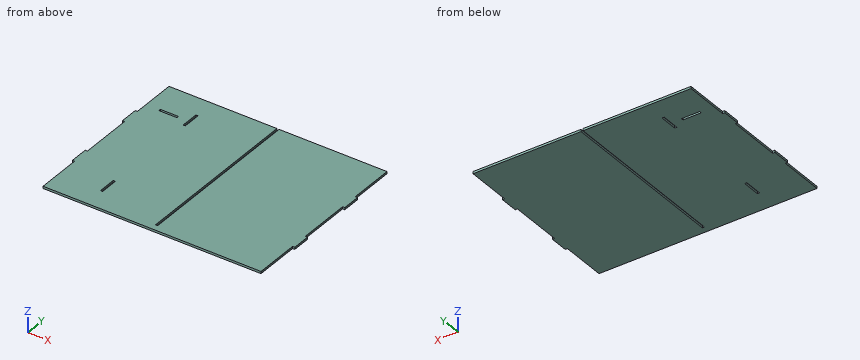
```python
from build123d import *

# Parameters (mm, degrees)
SKETCH1_W           = 6
SKETCH1_H           = 50
SKETCH1_W_2         = 50
SKETCH1_H_2         = 6
BOSS_EXTRUDE1_DEPTH = 6


with BuildPart() as part:
    # Sketch1 → Boss-Extrude1 (new body)
    with BuildSketch(Plane.XY):
        Polygon((0, 0), (297, 0), (297, -476), (303, -476), (303, 0), (600, 0), (600, -124), (606, -124), (606, -174), (600, -174), (600, -320), (606, -320), (606, -370), (600, -370), (600, -494), (0, -494), (0, -370), (-6, -370), (-6, -320), (0, -320), (0, -174), (-6, -174), (-6, -124), (0, -124), align=None)
        with Locations((119, -409)):
            Rectangle(SKETCH1_W, SKETCH1_H, mode=Mode.SUBTRACT)
        with Locations((119, -85)):
            Rectangle(SKETCH1_W, SKETCH1_H, mode=Mode.SUBTRACT)
        with Locations((62.5, -90.5)):
            Rectangle(SKETCH1_W_2, SKETCH1_H_2, mode=Mode.SUBTRACT)
    extrude(amount=BOSS_EXTRUDE1_DEPTH)


solid = part.part
```
Work out the finished part from the listing and answer in its coordinate system (mm). Round coordinates to 2 decimals unless told otherwise and drop trailing zeros. Loops run counter-clockwise (first coordinate to the right, second up) from the corner with the lowest first, then second, coordinate; pieces in that order, holes last. Notation, with made-up numbers: M 21,29.5 L 53,29.5 A17 ccw 53,48.5 Z; hole C 76.25,81.25 d4. An arc over 180 degrees is marked long. Use CSV: the item, a comma, the result in double quotes.
Q1. Section C-C, the plane z = 2.4 is taken. State how many separate pieces and enclosed holes the cut face has, then the cut area to 3 significant figures.
Determined:
separate pieces,"1"
enclosed holes,"3"
area,"294,000 mm2"
Q2. Consider L1, parallel to X at y = -390, z = 5; L2, parallel to X at y = -205.5, z = 2.6; L3, parallel to X at y = -92, z = 3.35. Determine where each line is inside the solid, lowest interval first.
Determined:
L1,"0 to 116, 122 to 297, 303 to 600"
L2,"0 to 297, 303 to 600"
L3,"0 to 37.5, 87.5 to 116, 122 to 297, 303 to 600"
Q3. Section B-B, the plane y = -220.5 is taken. Determine the outline of the cut face in (x, z).
Determined:
outline,"M 0,0 L 297,0 L 297,6 L 0,6 Z; M 303,0 L 600,0 L 600,6 L 303,6 Z"
Q4. Each of these flat-tipped pins is pushed along its axis until it touches: pin 1 (3 mm diameter, centred on y = -258.5, z = 2.5, fed in from +X); pin 2 (1 mm diameter, centred on x = 311, z = 2.5, fed in from +Y); pin 3 (1.5 mm diameter, centred on y = -298.5, z = 2.5, fed in from -X); pin 4 (1.8 mm diameter, centred on x = -2, z = 1.5, fed in from -Y). Where does it stop, or does it pass through?
Determined:
pin 1,"x = 600"
pin 2,"y = 0"
pin 3,"x = 0"
pin 4,"y = -370"
Q5. Section A-A, the plane y = -409.5 is taken. Determine the outline of the cut face in (x, z), then the cut area to 3 significant figures.
Determined:
outline,"M 0,0 L 116,0 L 116,6 L 0,6 Z; M 122,0 L 297,0 L 297,6 L 122,6 Z; M 303,0 L 600,0 L 600,6 L 303,6 Z"
area,"3,530 mm2"
